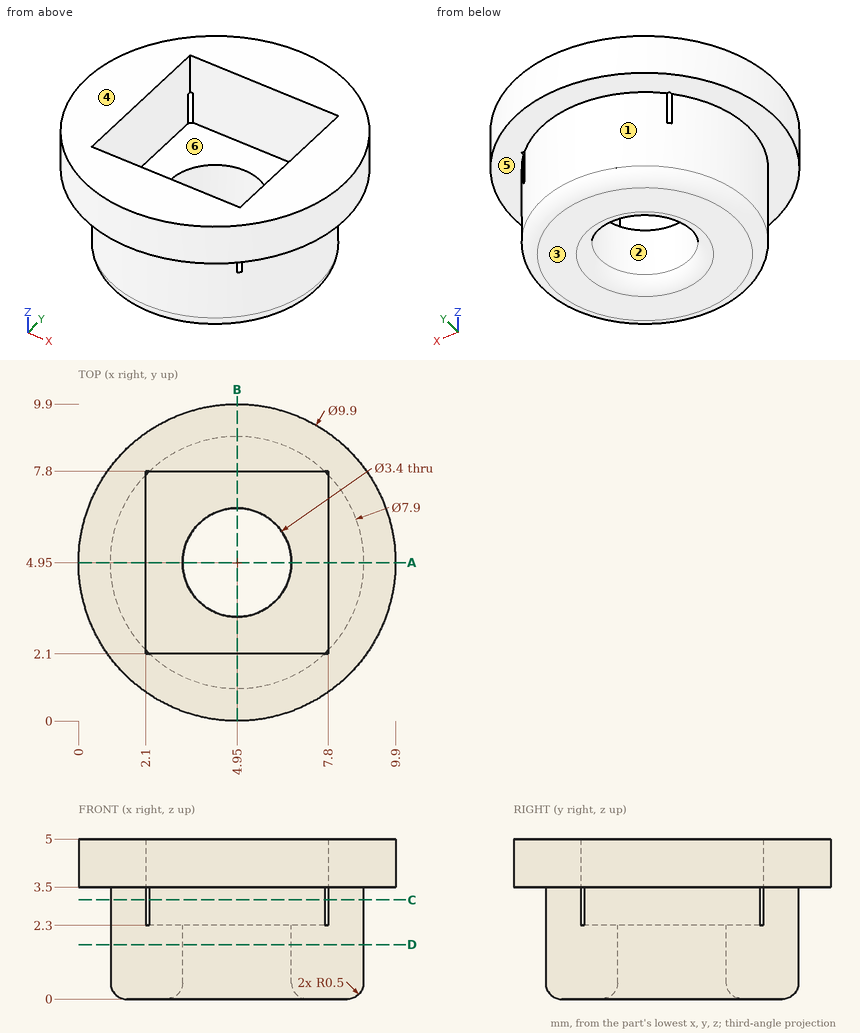
The figure shows three views and two pictorial views of one solid part (mm, origin at its lowest corner). Answer the questions. A direction names the side the tool comes from. Coordinates: 2 decimals unless noted, no trailing zeros. Loops run counter-clockwise (first coordinate to the right, second up) from the corner with the lowest first, then second, coordinate; pieces in that order, holes last.
(1) A tool of negligible diameter and unlimited length cuts with its end or side. For the marked faces 4, 5 and 6, from which of +Z, -Z, +X, -X, +Y, -Y can it reach the whole face along a straight path? Write none if from no direction.
Solution:
face 4: +Z, +X, -X, +Y, -Y
face 5: -Z
face 6: +Z
(2) Consider line 1 along Y through (x, z) = (4.95, 0.95); line 2 along Z through (x, y) = (9.25, 4.25). Determine where each line is inside the solid, lowest interval first.
Solution:
line 1: y = 1 to 3.25, 6.65 to 8.9
line 2: z = 3.5 to 5
(3) The part is cut by section D-D (z = 1.7). Determine the outline of the cut face in (x, y).
Solution:
outline: circle Ø7.9 at (4.95, 4.95); hole circle Ø3.4 at (4.95, 4.95)
(4) The mould has two halves that part along Y. Classify the marked faces 1, 2 and 3: released by +Y, released by -Y, zero draft, split by the parting line, or undercut.
Solution:
face 1: split by the parting line
face 2: undercut
face 3: zero draft
(5) The part is cut by section A-A (y = 4.95). Determine the outline of the cut face in (x, z).
Solution:
outline: (0, 3.5) - (1, 3.5) - (1, 0.5) arc R0.5 ccw to (1.5, 0) - (2.75, 0) arc R0.5 ccw to (3.25, 0.5) - (3.25, 2.3) - (2.1, 2.3) - (2.1, 5) - (0, 5) - close; (6.65, 0.5) arc R0.5 ccw to (7.15, 0) - (8.4, 0) arc R0.5 ccw to (8.9, 0.5) - (8.9, 3.5) - (9.9, 3.5) - (9.9, 5) - (7.8, 5) - (7.8, 2.3) - (6.65, 2.3) - close
(6) Flat-ended cylindrical pins translate along their axes: pin 1 Ø0.8 at (y, z) = (6.5, 4) entering from +X; pin 2 Ø4.5 at (x, y) = (4.5, 5.5) entering from +Z; pin 3 Ø1.5 at (x, z) = (4, 4) entering from -Y. Find the tip coordinate at first contact, or state that the pin passes through.
Solution:
pin 1: stops at x = 9.76
pin 2: stops at z = 2.3
pin 3: stops at y = 0
(7) The part is cut by section C-C (z = 3.1). Determine the outline of the cut face in (x, y), and give its area (3 significant figures).
Solution:
outline: (2.1, 2.22) - (2.1, 7.68) arc R3.95 ccw to start; (2.22, 2.1) arc R3.95 ccw to (7.68, 2.1) - close; (2.22, 7.8) - (7.68, 7.8) arc R3.95 ccw to start; (7.8, 2.22) arc R3.95 ccw to (7.8, 7.68) - close
area: 16.6 mm2
